Source: CAD feature listing. Evaluate the final solid. Frame: model axes, mm. A direction names the side the tool comes from. Give positions to 0.01 mm unless a question says otherwise; leave off trailing zeros. Order: outer loops, then holes, each group sorted by start corner. A loop starts at its lowest first (then second) coordinate and runs counter-clockwise, first axis right, second up. Notation, with made-up numbers: (87, -16.75) -> (133, -16.75) arc R26 cw to (133, 16.25) -> close; hole circle Ø5 at (69.25, -31.5). An arc over 180 degrees is marked (long way). Use CSV: the item, a comma, the result in double quotes.
```python
from build123d import *

# Parameters (mm, degrees)
SKETCH1_R           = 6
BOSS_EXTRUDE1_DEPTH = 15
SKETCH2_R           = 4
CUT_EXTRUDE1_DEPTH  = 16
SKETCH3_R           = 3
CUT_EXTRUDE2_DEPTH  = 16
CUT_EXTRUDE3_DEPTH  = 16
FILLET1_R           = 6
SKETCH5_R           = 7.5
BOSS_EXTRUDE2_DEPTH = 15
FILLET2_R           = 5


with BuildPart() as part:
    # Sketch1 → Boss-Extrude1 (new body)
    with BuildSketch(Plane(origin=(0, 0, 0), x_dir=(0, 0, -1), z_dir=(1, 0, 0))):
        with BuildLine():
            ThreePointArc((24.992781164, -0.60074095), (9.243822678, 113.703988064), (-41.858816097, 217.155044504))
            Line((-41.858816097, 217.155044504), (-48.12160564, 172.59298141))
            ThreePointArc((-48.12160564, 172.59298141), (-22.274376436, 90.661190514), (-24.538993202, 4.778892408))
            ThreePointArc((-24.538993202, 4.778892408), (2.400538477, 24.88448141), (25, 0))
            ThreePointArc((25, 0), (24.998195226, -0.30039216), (24.992781164, -0.60074095))
        make_face()
        with BuildLine():
            ThreePointArc((-24.538993202, 4.778892408), (-2.699369305, -24.853840857), (24.992781164, -0.60074095))
            ThreePointArc((24.992781164, -0.60074095), (24.998195226, -0.30039216), (25, 0))
            ThreePointArc((25, 0), (2.400538477, 24.88448141), (-24.538993202, 4.778892408))
        make_face()
        with Locations((0, -12)):
            Circle(SKETCH1_R, mode=Mode.SUBTRACT)
    extrude(amount=BOSS_EXTRUDE1_DEPTH)

    # Sketch2 → Cut-Extrude1 (cut, through all)
    with BuildSketch(Plane(origin=(15, 0, 0), x_dir=(0, 0, -1), z_dir=(1, 0, 0))):
        with Locations((0, 28)):
            Circle(SKETCH2_R)
    extrude(amount=-CUT_EXTRUDE1_DEPTH, mode=Mode.SUBTRACT)

    # Sketch3 → Cut-Extrude2 (cut, through all)
    with BuildSketch(Plane(origin=(15, 0, 0), x_dir=(0, 0, -1), z_dir=(1, 0, 0))):
        with Locations((-40.714528231, 175)):
            Circle(SKETCH3_R)
        with Locations((-37.235200707, 199.756701719)):
            Circle(SKETCH3_R)
    extrude(amount=-CUT_EXTRUDE2_DEPTH, mode=Mode.SUBTRACT)

    # Sketch4 → Cut-Extrude3 (cut, through all)
    with BuildSketch(Plane(origin=(15, 0, 0), x_dir=(0, 0, -1), z_dir=(1, 0, 0))):
        with BuildLine():
            ThreePointArc((-11.749836025, 155.008629259), (-20.960958666, 173.77628952), (-31.260870979, 191.969190837))
            Line((-31.260870979, 191.969190837), (-35.976814508, 158.413509038))
            Line((-35.976814508, 158.413509038), (-11.749836025, 155.008629259))
        make_face()
        with BuildLine():
            Line((-9.354323007, 149.622823998), (-33.760235475, 153.052851308))
            ThreePointArc((-33.760235475, 153.052851308), (-24.416431689, 125.419954523), (-18.166319592, 96.927503721))
            Line((-18.166319592, 96.927503721), (-9.354323007, 149.622823998))
        make_face()
        with BuildLine():
            ThreePointArc((14.161868129, 72.691486719), (5.930300275, 107.334766496), (-5.730334656, 140.979158838))
            Line((-5.730334656, 140.979158838), (-15.958464631, 79.815428272))
            Line((-15.958464631, 79.815428272), (14.161868129, 72.691486719))
        make_face()
        with BuildLine():
            Line((15.468075791, 65.189422352), (-15.356589243, 72.479949778))
            ThreePointArc((-15.356589243, 72.479949778), (-14.750380465, 52.717361117), (-15.619336812, 32.964581198))
            Line((-15.619336812, 32.964581198), (15.468075791, 65.189422352))
        make_face()
        with BuildLine():
            ThreePointArc((19.721068997, 24.377203305), (18.614609922, 40.455333735), (16.779570125, 56.466678425))
            Line((16.779570125, 56.466678425), (-2, 37))
            ThreePointArc((-2, 37), (10.561248293, 33.615157675), (19.721068997, 24.377203305))
        make_face()
    extrude(amount=-CUT_EXTRUDE3_DEPTH, mode=Mode.SUBTRACT)

    # Fillet1
    fillet1_edges = [part.edges().sort_by_distance(p)[0] for p in [
        (7.5, 155.008629259, 11.749836025),
        (7.5, 158.413509038, 35.976814508),
        (7.5, 191.969190837, 31.260870979),
        (7.5, 96.927503721, 18.166319592),
        (7.5, 153.052851308, 33.760235475),
        (7.5, 149.622823998, 9.354323007),
        (7.5, 72.691486719, -14.161868129),
        (7.5, 79.815428272, 15.958464631),
        (7.5, 140.979158838, 5.730334656),
        (7.5, 32.964581198, 15.619336812),
        (7.5, 72.479949778, 15.356589243),
        (7.5, 65.189422352, -15.468075791),
        (7.5, 24.377203305, -19.721068997),
        (7.5, 37, 2),
        (7.5, 56.466678425, -16.779570125),
    ]]
    fillet(fillet1_edges, radius=FILLET1_R)

    # Sketch5 → Boss-Extrude2 (add)
    with BuildSketch(Plane(origin=(15, 0, 0), x_dir=(0, 0, -1), z_dir=(1, 0, 0))):
        with BuildLine():
            ThreePointArc((-34, -9), (-28.696699141, -11.196699141), (-26.5, -16.5))
            ThreePointArc((-26.5, -16.5), (-28.087357429, -21.114180081), (-32.177508753, -23.775199355))
            ThreePointArc((-32.177508753, -23.775199355), (-19.40613231, -22.280390349), (-6.675855702, -24.092176129))
            ThreePointArc((-6.675855702, -24.092176129), (-19.898447082, -15.134457497), (-25, 0))
            ThreePointArc((-25, 0), (-27.636038969, -6.363961031), (-34, -9))
        make_face()
        with Locations((-34, -16.5)):
            Circle(SKETCH5_R)
    extrude(amount=-BOSS_EXTRUDE2_DEPTH)

    # Fillet2
    fillet2_edges = [part.edges().sort_by_distance(p)[0] for p in [
        (7.5, 172.59298141, 48.12160564),
        (7.5, 217.155044504, 41.858816097),
    ]]
    fillet(fillet2_edges, radius=FILLET2_R)


solid = part.part
```
1. Section query D-D on y = 28. Return loops of the section in (x, z), plus the area to 3 significant figures.
Answer below:
outline,"(0, -24.54) -> (15, -24.54) -> (15, -4) -> (0, -4) -> close; (0, 4) -> (15, 4) -> (15, 21.1) -> (0, 21.1) -> close"
area,"565 mm²"
2. Access query for faces 5 (the cylindrical face through (7.4, 148.14, 11.49)), 6 (the cylindrical face through (7.605, 208.616, 39.716)), 7 (the cylindrical face through (7.605, -6.294, 27.566)). Directions: +Z, -Z, +X, -X, +Y, -Y. A direction counts if a zero-diameter tool reaches every point of the face in a straight line with its end or side. Return the directions, or none.
Answer below:
face 5,"+X, -X"
face 6,"+X, -X, +Y"
face 7,"+Z, +X, -X"
3. Section query A-A on y = 94.5. Return loops of the section in (x, z).
Answer below:
outline,"(0, -14.56) -> (15, -14.56) -> (15, -9.41) -> (0, -9.41) -> close; (0, 13.5) -> (15, 13.5) -> (15, 22.84) -> (0, 22.84) -> close"
4. Ray query, line 1 along Y through (x, z) = (2.25, 7.5); line 2 along Z through (x, y) = (10.5, 175); line 3 along Z through (x, y) = (4.5, 105). Return the intervals inside material, ascending.
Answer below:
line 1,"y = -23.87 to 42.81, 70.62 to 77.81, 122.15 to 157.74"
line 2,"z = 15.96 to 21.61, 33.63 to 37.71, 43.71 to 47.78"
line 3,"z = -11.8 to -6.6, 11.75 to 24.7"
5. Section query B-B on z = 0. Return loops of the section in (x, y).
Answer below:
outline,"(0, -25) -> (15, -25) -> (15, -18) -> (0, -18) -> close; (0, -6) -> (15, -6) -> (15, 24) -> (0, 24) -> close; (0, 32) -> (15, 32) -> (15, 49.16) -> (0, 49.16) -> close; (0, 68.85) -> (15, 68.85) -> (15, 76.04) -> (0, 76.04) -> close; (0, 122.46) -> (15, 122.46) -> (15, 140.11) -> (0, 140.11) -> close"
6. Section query C-C on z = 28. Return loops of the section in (x, y), plus the area to 3 significant figures.
Answer below:
outline,"(0, -22.92) -> (15, -22.92) -> (15, -6.71) -> (0, -6.71) -> close; (0, 119.48) -> (15, 119.48) -> (15, 137.24) -> (0, 137.24) -> close; (0, 150.62) -> (15, 150.62) -> (15, 157.29) -> (0, 157.29) -> close; (0, 179.77) -> (15, 179.77) -> (15, 196.23) -> (0, 196.23) -> close"
area,"857 mm²"
7. Pin query (flat end, axial travel): P1, Ø8, axis at x = 9.5, z = 28, coming from the +Y side; P2, Ø5.5, axis at y = 175, z = 40.71, coming from the +X side; P3, Ø3, axis at x = 12, y = 167, coming from the -Z side; P4, Ø1.5, axis at x = 8.5, y = 168.5, coming from the -Z side. Return the tip coordinate at first contact, or that it passes through.
Answer below:
P1,"stops at y = 202.6"
P2,"passes through"
P3,"stops at z = 11.16"
P4,"stops at z = 12.26"
8. Mould query, pull axis Z, two halves, no side actions, for faces 1 (the cylindrical face through (7.395, 39.5, -3.963)), 2 (the cylindrical face through (7.4, -6.05, 0.78)), 3 (the cylindrical face through (7.4, 106.02, -11.51)), 4 (the cylindrical face through (7, -20, -15)). Classes: released by +Z, released by -Z, zero draft, split by the parting line, or undercut.
Answer below:
face 1,"undercut"
face 2,"undercut"
face 3,"released by -Z"
face 4,"split by the parting line"
